Can you work these out from the model? Positions are in its coordinate system, mm. Face numbers are marked on the shaded views. A direction names the side the tool comes from. Coordinates: 2 decimals unless noted, no trailing zeros. Order: outer loops, then holes, each group sorted by start corner. A loop starts at its lowest first (then second) coordinate and runs counter-clockwise, first axis right, second up. Notation, with made-up numbers: (15, 59) -> (65, 59) arc R17 cw to (65, 69) -> close; hole circle Ø11 at (81.25, 6.25). An arc over 180 degrees is marked (long way). Write item = value, one per line.
```python
from build123d import *

# Parameters (mm, degrees)
SKETCH_1_W             = 200
SKETCH_1_H             = 100
EXTRUDE_1_DEPTH        = 2
SKETCH_2_W             = 200
SKETCH_2_H             = 100
SKETCH_2_W_2           = 196
SKETCH_2_H_2           = 96
EXTRUDE_2_DEPTH        = 63
SKETCH_3_W             = 7
SKETCH_3_H             = 18
CUT_EXTRUDE_1_DEPTH    = 63
SKETCH_4_W             = 200
SKETCH_4_H             = 15
EXTRUDE_3_DEPTH        = 3
EXTRUDE_4_DEPTH        = 5
PATTERN_LINEAR_1_COUNT = 2
PATTERN_LINEAR_1_PITCH = 80
PATTERN_LINEAR_2_COUNT = 2
PATTERN_LINEAR_2_PITCH = 80
SKETCH_6_R             = 2
CUT_EXTRUDE_2_DEPTH    = 5
FILLET_1_R             = 1
SKETCH_7_W             = 50
SKETCH_7_H             = 25
CUT_EXTRUDE_3_DEPTH    = 281


with BuildPart() as part:
    # 草图1 → 凸台-拉伸1 (new body)
    with BuildSketch(Plane.XY):
        Rectangle(SKETCH_1_W, SKETCH_1_H)
    extrude(amount=EXTRUDE_1_DEPTH)

    # 草图2 → 凸台-拉伸2 (add)
    with BuildSketch(Plane.XY.offset(2)):
        Rectangle(SKETCH_2_W, SKETCH_2_H)
        Rectangle(SKETCH_2_W_2, SKETCH_2_H_2, mode=Mode.SUBTRACT)
    extrude(amount=EXTRUDE_2_DEPTH)

    # 草图3 → 切除-拉伸1 (cut)
    with BuildSketch(Plane(origin=(0, 0, 0), x_dir=(-1, 0, 0), z_dir=(0, 0, -1))):
        with Locations((12.5, 0)):
            Rectangle(SKETCH_3_W, SKETCH_3_H)
        with Locations((-12.5, 0)):
            Rectangle(SKETCH_3_W, SKETCH_3_H)
    extrude(amount=-CUT_EXTRUDE_1_DEPTH, mode=Mode.SUBTRACT)

    # 草图4 → 凸台-拉伸3 (add)
    with BuildSketch(Plane.XY.offset(65)):
        with Locations((0, 57.5)):
            Rectangle(SKETCH_4_W, SKETCH_4_H)
        with Locations((0, -57.5)):
            Rectangle(SKETCH_4_W, SKETCH_4_H)
    extrude(amount=-EXTRUDE_3_DEPTH)

    # 草图5 → 凸台-拉伸4 (add)
    with BuildSketch(Plane(origin=(0, 0, 0), x_dir=(0, 0, -1), z_dir=(1, 0, 0))):
        Polygon((-62, 60), (-52, 50), (-62, 50), align=None)
        Polygon((-52, -50), (-62, -50), (-62, -60), align=None)
    extrude_4 = extrude(amount=EXTRUDE_4_DEPTH)

    # 阵列(线性)1: 凸台-拉伸4 ×2
    with Locations(*[(-i * PATTERN_LINEAR_1_PITCH, 0, 0) for i in range(1, PATTERN_LINEAR_1_COUNT)]):
        add(extrude_4)

    # 阵列(线性)2: 凸台-拉伸4 ×2
    with Locations(*[(i * PATTERN_LINEAR_2_PITCH, 0, 0) for i in range(1, PATTERN_LINEAR_2_COUNT)]):
        add(extrude_4)

    # 草图6 → 切除-拉伸2 (cut)
    with BuildSketch(Plane(origin=(0, 0, 62), x_dir=(-1, 0, 0), z_dir=(0, 0, -1))):
        with Locations((-40, -57.5)):
            Circle(SKETCH_6_R)
        with Locations(Location((40, -57.5, 0), (0, 0, 180))):
            Circle(SKETCH_6_R)
        with Locations((40, 57.5)):
            Circle(SKETCH_6_R)
        with Locations(Location((-40, 57.5, 0), (0, 0, 180))):
            Circle(SKETCH_6_R)
    extrude(amount=-CUT_EXTRUDE_2_DEPTH, mode=Mode.SUBTRACT)

    # 圆角1
    fillet_1_edges = [part.edges().sort_by_distance(p)[0] for p in [
        (42.5, 50, 62),
        (-37.5, -50, 62),
        (-37.5, 50, 62),
        (92.5, 50, 62),
        (42.5, -50, 62),
        (0, 48, 65),
        (0, -48, 65),
        (92.5, -50, 62),
    ]]
    fillet(fillet_1_edges, radius=FILLET_1_R)

    # 草图7 → 切除-拉伸3 (cut)
    with BuildSketch(Plane(origin=(100, 0, 0), x_dir=(0, 0, -1), z_dir=(1, 0, 0))):
        with Locations((-40, 0)):
            Rectangle(SKETCH_7_W, SKETCH_7_H)
    extrude(amount=-CUT_EXTRUDE_3_DEPTH, mode=Mode.SUBTRACT)


solid = part.part
```
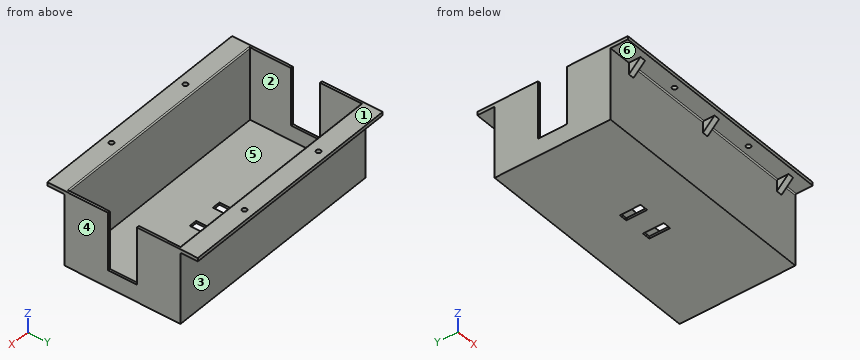
Item 1: I want a section at C-C, the plane z = 22. Please give me the cut outline in (x, y), plus the area to 3 significant figures.
A:
outline = (-100, -50) -> (100, -50) -> (100, -12.5) -> (98, -12.5) -> (98, -48) -> (-98, -48) -> (-98, -12.5) -> (-100, -12.5) -> close; (-100, 12.5) -> (-98, 12.5) -> (-98, 48) -> (98, 48) -> (98, 12.5) -> (100, 12.5) -> (100, 50) -> (-100, 50) -> close
area = 1,080 mm2
Item 2: For the marked faces 4, 5 and 6, which set-ups out of +Z, -Z, +X, -X, +Y, -Y let a thin tool reach every point of the face, with its end or its side?
A:
face_4 = +Z, -Z, +X, +Y, -Y
face_5 = +Z
face_6 = -Z, -Y
Item 3: If I drill on probe 1 along Y at (x, z) = (-40, 63.8); probe 2 along X at (y, z) = (-18.5, 61.5); probe 3 along Y at (x, z) = (-84.5, 22), over which ranges is the centre line in solid material (lowest first)?
A:
probe_1 = -65 to -59.5, -55.5 to -48, 48 to 55.5, 59.5 to 65
probe_2 = -100 to -98, 98 to 100
probe_3 = -50 to -48, 48 to 50
Item 4: I want a section at D-D, the plane y = -35.5. Please give me the cut outline in (x, z).
A:
outline = (-100, 0) -> (100, 0) -> (100, 65) -> (98, 65) -> (98, 2) -> (-98, 2) -> (-98, 65) -> (-100, 65) -> close
Item 5: I want a section at B-B, the plane x = -40. Please give me the cut outline in (y, z), plus the area to 3 significant figures.
A:
outline = (-65, 62) -> (-59.5, 62) -> (-59.5, 65) -> (-65, 65) -> close; (-55.5, 62) -> (-51, 62) arc R1 cw to (-50, 61) -> (-50, 0) -> (50, 0) -> (50, 61) arc R1 cw to (51, 62) -> (55.5, 62) -> (55.5, 65) -> (49, 65) arc R1 ccw to (48, 64) -> (48, 2) -> (-48, 2) -> (-48, 64) arc R1 ccw to (-49, 65) -> (-55.5, 65) -> close; (59.5, 62) -> (65, 62) -> (65, 65) -> (59.5, 65) -> close
area = 518 mm2
Item 6: I want a section at A-A, the plane y = 2. Please give me the cut outline in (x, z).
A:
outline = (-100, 0) -> (-16, 0) -> (-16, 2) -> (-98, 2) -> (-98, 15) -> (-100, 15) -> close; (-9, 0) -> (9, 0) -> (9, 2) -> (-9, 2) -> close; (16, 0) -> (100, 0) -> (100, 15) -> (98, 15) -> (98, 2) -> (16, 2) -> close
Item 7: I'm going to push flat-ended pins straight in: P1, Ø0.6, axis at x = -99.5, y = 1.5, coming from the +Z side; P2, Ø2, axis at x = 14, z = 1.5, coming from the -Y side; P3, Ø12, axis at x = 36, y = -32.5, coming from the +Z side; P4, Ø3.5, axis at x = -40, y = 57.5, coming from the -Z side. Where does each tip first touch, or does it pass through?
A:
P1 = 15
P2 = -50
P3 = 2
P4 = through
Item 8: If we mould it in two halves opening along Y, with no side actions, what happens to the marked faces 1, 2 and 3? For each: pulls with the +Y half, pulls with the -Y half, needs draft (parallel to the pull), parting line crosses it, or undercut.
A:
face_1 = needs draft
face_2 = undercut
face_3 = pulls with the +Y half
